from build123d import *

# Parameters (mm, degrees)
F0_R     = 11.684
F0_R_2   = 9.40435
F0_R_3   = 7.8867
F1_DEPTH = 4.826
F2_DEPTH = 17.526
F3_SIZE  = 0.762
F4_SIZE  = 0.254


with BuildPart() as f1:
    # F0 (on Right) → F1 (new body)
    with BuildSketch(Plane.YZ):
        Circle(F0_R)
        Circle(F0_R_2, mode=Mode.SUBTRACT)
        Circle(F0_R_2)
        Circle(F0_R_3, mode=Mode.SUBTRACT)
    extrude(amount=F1_DEPTH)

    # F0 (on Right) → F2 (join)
    with BuildSketch(Plane.YZ):
        Circle(F0_R_2)
        Circle(F0_R_3, mode=Mode.SUBTRACT)
    extrude(amount=-F2_DEPTH)

    # F3
    f3_edges = [f1.edges().sort_by_distance(p)[0] for p in [
        (4.826, -11.684, 0),
    ]]
    chamfer(f3_edges, length=F3_SIZE)

    # F4
    f4_edges = [f1.edges().sort_by_distance(p)[0] for p in [
        (-17.526, -9.40435, 0),
    ]]
    chamfer(f4_edges, length=F4_SIZE)


solid = f1.part
Geometry: final body of the model. Coordinates: model frame, mm. A direction names the side the tool comes from. Give positions to 0.01 mm unless a question says otherwise; leave off trailing zeros. Loops run counter-clockwise (first coordinate to the right, second up) from the corner with the lowest first, then second, coordinate; pieces in that order, holes last. Notation, with made-up numbers: M 85,30.5 L 114,30.5 A28 ccw 114,61.5 Z; hole C 58.5,78 d5. An arc over 180 degrees is marked long. Put each result on its own line as item: value. Start each with the question number.
1) Access query for faces 1 (the flat face through (0, 1, 10)), 2 (the flat face through (4.826, 6, 6)). Directions: +Z, -Z, +X, -X, +Y, -Y. A direction counts if a zero-diameter tool reaches every point of the face in a straight line with its end or side. Return the directions, or none.
2) Cut plane C-C (x = -1.5). Output: boundary loops of the cut face in (y, z).
3) Pull-direction query (Z, two-part tool) for faces 3 (the cylindrical face through (-8.52, -2.04, -9.18)), 4 (the flat face through (-17.526, 4, 7)), 5 (the cylindrical face through (-6.5, -1.7, -7.7)); classes: pulls with the +Z half, pulls with the -Z half, needs draft (parallel to the pull), parting line crosses it, or undercut.
4) Cut plane A-A (y = 0). Output: boundary loops of the cut face in (x, z), then the cut area to 3 significant figures.
5) Ray query, line 1 along Z through (x, y) = (-0.75, 0); line 2 along Y through (x, z) = (-6.25, -5.5); line 3 along Y through (x, z) = (-10.5, 2). Return the intervals inside material, ascending.
6) Contact query for flat-ended pins moving along their axis: pin 1 (1.5 mm diameter, centred on x = -0.5, z = -4.5, fed in from +Y); pin 2 (8 mm diameter, centred on x = -0.5, z = -4.5, fed in from -Y); pin 3 (12 mm diameter, centred on x = -10.5, y = 9, fed in from +Z). Output: stop coordinate, or through.
Verdict:
1. face 1: -X
1. face 2: +Z, -Z, +X, +Y, -Y
2. outline: C 0,0 d18.81; hole C 0,0 d15.77
3. face 3: parting line crosses it
3. face 4: needs draft
3. face 5: undercut
4. outline: M -17.53,-9.15 L -17.27,-9.4 L 0,-9.4 L 0,-11.68 L 4.06,-11.68 L 4.83,-10.92 L 4.83,-7.89 L -17.53,-7.89 Z; M -17.53,7.89 L 4.83,7.89 L 4.83,10.92 L 4.06,11.68 L 0,11.68 L 0,9.4 L -17.27,9.4 L -17.53,9.15 Z
4. area: 89.2 mm2
5. line 1: -9.4 to -7.89, 7.89 to 9.4
5. line 2: -7.63 to -5.65, 5.65 to 7.63
5. line 3: -9.19 to -7.63, 7.63 to 9.19
6. pin 1: y = 11
6. pin 2: y = -11.67
6. pin 3: z = 8.91
